Check sheet for the modelled part. Datum: model origin and axes. Units: mm. Face numbers are marked on the shaded views. A direction names the side the tool comes from. Round coordinates to 2 decimals unless told otherwise and drop trailing zeros. Loops run counter-clockwise (first coordinate to the right, second up) from the corner with the lowest first, then second, coordinate; pieces in that order, holes last. Notation, with made-up numbers: (78, 82) -> (103, 82) arc R19 ccw to (103, 113) -> close; hole circle Ø10 at (51, 42.25). An arc over 180 degrees is marked (long way). One line per question, with ' | ' between items.
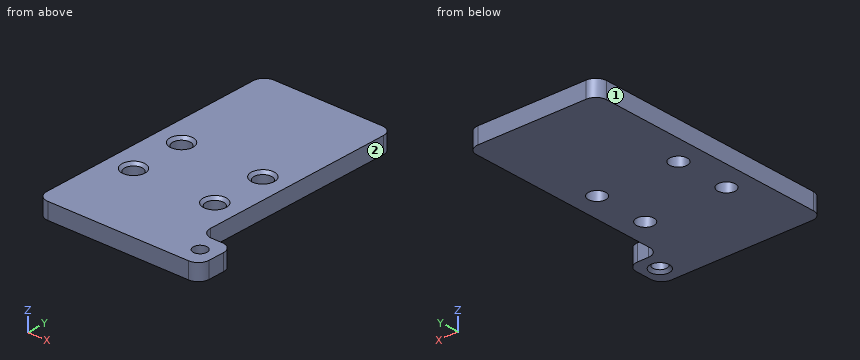
```python
from build123d import *

# Parameters (mm, degrees)
SKETCH_1_R      = 1.6
SKETCH_1_R_2    = 1.25
EXTRUDE_1_DEPTH = 3
CHAMFER_1_SIZE  = 0.5
FILLET_1_R      = 2


with BuildPart() as part:
    # 草图1 → 凸台-拉伸1 (new body)
    with BuildSketch(Plane.XY):
        Polygon((12, -25), (18, -25), (18, -32), (-12, -32), (-12, 15), (12, 15), align=None)
        with Locations((-7.5, -7)):
            Circle(SKETCH_1_R, mode=Mode.SUBTRACT)
        with Locations((7.5, -7)):
            Circle(SKETCH_1_R, mode=Mode.SUBTRACT)
        with Locations((-7.5, -17)):
            Circle(SKETCH_1_R, mode=Mode.SUBTRACT)
        with Locations((7.5, -17)):
            Circle(SKETCH_1_R, mode=Mode.SUBTRACT)
        with Locations((15, -28.5)):
            Circle(SKETCH_1_R_2, mode=Mode.SUBTRACT)
    extrude(amount=EXTRUDE_1_DEPTH)

    # 倒角1
    chamfer_1_edges = [part.edges().sort_by_distance(p)[0] for p in [
        (13.75, -28.5, 0),
        (-9.1, -7, 3),
        (5.9, -7, 3),
        (-9.1, -17, 3),
        (5.9, -17, 3),
    ]]
    chamfer(chamfer_1_edges, length=CHAMFER_1_SIZE)

    # 圆角1
    fillet_1_edges = [part.edges().sort_by_distance(p)[0] for p in [
        (-12, -32, 1.5),
        (-12, 15, 1.5),
        (12, 15, 1.5),
        (12, -25, 1.5),
        (18, -25, 1.5),
        (18, -32, 1.5),
    ]]
    fillet(fillet_1_edges, radius=FILLET_1_R)


solid = part.part
```
(1) Sectioned sample at A-A, the plane x = 7.5. Record the cut outline in (y, z).
Answer:
outline: (-32, 0) -> (-18.6, 0) -> (-18.6, 2.5) -> (-19.1, 3) -> (-32, 3) -> close; (-15.4, 0) -> (-8.6, 0) -> (-8.6, 2.5) -> (-9.1, 3) -> (-14.9, 3) -> (-15.4, 2.5) -> close; (-5.4, 0) -> (15, 0) -> (15, 3) -> (-4.9, 3) -> (-5.4, 2.5) -> close
(2) Sectioned sample at B-B, the plane y = -7. Record the cut outline in (x, z).
Answer:
outline: (-12, 0) -> (-9.1, 0) -> (-9.1, 2.5) -> (-9.6, 3) -> (-12, 3) -> close; (-5.9, 0) -> (5.9, 0) -> (5.9, 2.5) -> (5.4, 3) -> (-5.4, 3) -> (-5.9, 2.5) -> close; (9.1, 0) -> (12, 0) -> (12, 3) -> (9.6, 3) -> (9.1, 2.5) -> close
(3) Sectioned sample at D-D, the plane z = 1.15. Record the cut outline in (x, y), and give its area (3 significant figures).
Answer:
outline: (-12, -30) arc R2 ccw to (-10, -32) -> (16, -32) arc R2 ccw to (18, -30) -> (18, -27) arc R2 ccw to (16, -25) -> (14, -25) arc R2 cw to (12, -23) -> (12, 13) arc R2 ccw to (10, 15) -> (-10, 15) arc R2 ccw to (-12, 13) -> close; hole circle Ø3.2 at (-7.5, -17); hole circle Ø3.2 at (-7.5, -7); hole circle Ø3.2 at (7.5, -17); hole circle Ø3.2 at (7.5, -7); hole circle Ø2.5 at (15, -28.5) | area: 1,130 mm2
(4) Sectioned sample at C-C, the plane x = 15. Record the cut outline in (y, z).
Answer:
outline: (-32, 0) -> (-30.25, 0) -> (-29.75, 0.5) -> (-29.75, 3) -> (-32, 3) -> close; (-27.25, 0.5) -> (-26.75, 0) -> (-25, 0) -> (-25, 3) -> (-27.25, 3) -> close
(5) Set-up check for the marked faces 1 and 2: record each of +Z, -Z, +X, -X, +Y, -Y from which the full face is reachable in a straight line by a thin tool's end or side.
Answer:
face 1: +Z, -Z, -X, +Y, -Y | face 2: +Z, -Z, +X, +Y
(6) Scan lines: probe 1 along Y at (x, z) = (-7.5, 1.05); probe 2 along Y at (x, z) = (-8.5, 1.1); probe 3 along Y at (x, z) = (15, 1.6). Record each from-to range of solid material in increasing order.
Answer:
probe 1: y = -32 to -18.6, -15.4 to -8.6, -5.4 to 15 | probe 2: y = -32 to -18.25, -15.75 to -8.25, -5.75 to 15 | probe 3: y = -32 to -29.75, -27.25 to -25
(7) Go/stop test with flat-tipped pins: pin 1 (1 mm diameter, centred on y = -6.5, z = 2.5, fed in from +X); pin 2 (4 mm diameter, centred on x = -7.5, y = -17, fed in from +Z); pin 3 (0.6 mm diameter, centred on x = 15.5, z = 1.5, fed in from +Y). Record where each tip stops, or that it passes through.
Answer:
pin 1: stops at x = 12 | pin 2: stops at z = 2.9 | pin 3: stops at y = -25
